```python
from build123d import *

# Parameters (mm, degrees)
SKETCH2_W           = 15.1
SKETCH2_H           = 3.1
BOSS_EXTRUDE2_DEPTH = 3


with BuildPart() as part:
    # Sketch2 → Boss-Extrude2 (new body)
    with BuildSketch(Plane(origin=(0, 0, 0), x_dir=(1, 0, 0), z_dir=(0, 1, 0))):
        with BuildLine():
            Line((0, 0), (109.814085495, 0))
            ThreePointArc((109.814085495, 0), (146.05, 60.93), (182.285914505, 0))
            Line((182.285914505, 0), (200, 0))
            Line((200, 0), (200, 70))
            Line((200, 70), (170, 90))
            Line((170, 90), (0, 90))
            Line((0, 90), (0, 0))
        make_face()
        with Locations((21.82, 32.29)):
            Rectangle(SKETCH2_W, SKETCH2_H, mode=Mode.SUBTRACT)
        with Locations((65.47, 32.29)):
            Rectangle(SKETCH2_W, SKETCH2_H, mode=Mode.SUBTRACT)
        with Locations((21.82, 65.29)):
            Rectangle(SKETCH2_W, SKETCH2_H, mode=Mode.SUBTRACT)
        with Locations((65.47, 65.29)):
            Rectangle(SKETCH2_W, SKETCH2_H, mode=Mode.SUBTRACT)
        with Locations((134.54, 65.29)):
            Rectangle(SKETCH2_W, SKETCH2_H, mode=Mode.SUBTRACT)
        with Locations((178.19, 65.29)):
            Rectangle(SKETCH2_W, SKETCH2_H, mode=Mode.SUBTRACT)
    extrude(amount=BOSS_EXTRUDE2_DEPTH)


solid = part.part
```
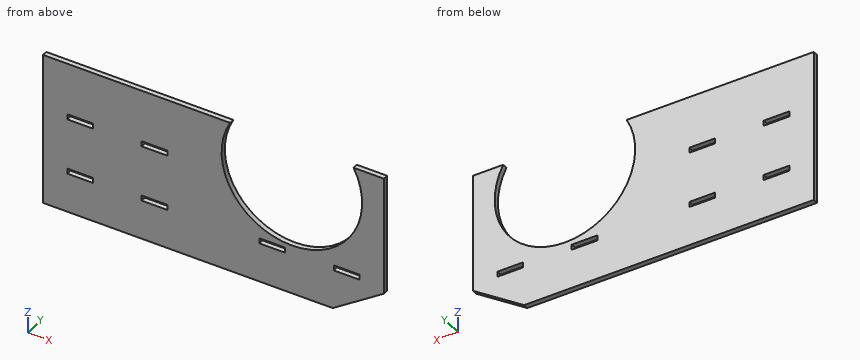
Here's how the part is built. I have some questions about the finished solid (model axes, mm). Give positions to 0.01 mm unless a question says otherwise; leave off trailing zeros. Write each loop counter-clockwise with the first axis right and the second up, starting at its lowest first coordinate (ties: lowest second). Pieces come first, ordered by that corner, then holes. Notation, with made-up numbers: (-9.75, 55.5) -> (43.25, 55.5) arc R12 ccw to (43.25, 61.5) -> close; hole circle Ø10 at (4.25, -34.75). An arc over 180 degrees is marked (long way). Use one line per item in the form item = value.
1) If I drill on L1, parallel to Z at x = 29, y = 2.15; L2, parallel to X at y = 1.5, z = -19.69; L3, parallel to Z at x = 108, y = 1.25, over which ranges is the centre line in solid material (lowest first)? Write a range as [from, to].
Verdict:
L1 = [-90, -66.84], [-63.74, -33.84], [-30.74, 0]
L2 = [0, 104.81], [187.29, 200]
L3 = [-90, -35.59], [-3.79, 0]
2) Suppose I cut it at B-B (z = -19.69). Please give me the cut outline in (x, y), and give its area (3 significant figures).
Verdict:
outline = (0, 0) -> (104.81, 0) -> (104.81, 3) -> (0, 3) -> close; (187.29, 0) -> (200, 0) -> (200, 3) -> (187.29, 3) -> close
area = 353 mm2
3) Suppose I cut it at D-D (x = 146.05). Please give me the cut outline in (y, z).
Verdict:
outline = (0, -90) -> (3, -90) -> (3, -60.93) -> (0, -60.93) -> close
4) I'm going to push a flat-ended pin straight in: pin 1 (1.5 mm diameter, centred on x = 146, y = 1.5, fed in from +Z). Where does the tip first touch, or does it pass through?
Verdict:
pin_1 = -60.92
5) Suppose I cut it at A-A (x = 70.5). Please give me the cut outline in (y, z), and give its area (3 significant figures).
Verdict:
outline = (0, -90) -> (3, -90) -> (3, -66.84) -> (0, -66.84) -> close; (0, -63.74) -> (3, -63.74) -> (3, -33.84) -> (0, -33.84) -> close; (0, -30.74) -> (3, -30.74) -> (3, 0) -> (0, 0) -> close
area = 251 mm2
6) Suppose I cut it at C-C (y = 2.35). Give the number of separate pieces and of enclosed holes in the cut face, and give its area (3 significant figures).
Verdict:
separate_pieces = 1
enclosed_holes = 6
area = 13,200 mm2
